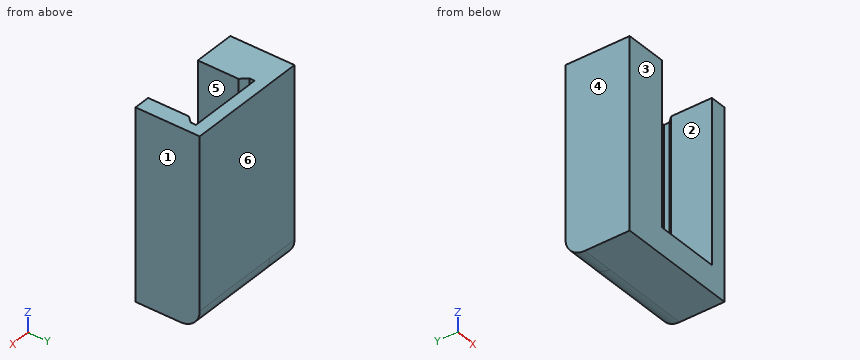
from build123d import *

# Parameters (mm, degrees)
SKETCH_1_W          = 29.5
SKETCH_1_H          = 10
EXTRUDE_1_DEPTH     = 13.06
FILLET_1_R          = 3
CUT_EXTRUDE_1_DEPTH = 25.35
EXTRUDE_START       = 1
EXTRUDE_2_DEPTH     = 1
EXTRUDE_START_2     = -13.06
EXTRUDE_3_DEPTH     = 5


with BuildPart() as part:
    # 草图1 → 凸台-拉伸1 (new body)
    with BuildSketch(Plane(origin=(0, 0, 0), x_dir=(0, 0, -1), z_dir=(1, 0, 0))):
        Rectangle(SKETCH_1_W, SKETCH_1_H)
    extrude(amount=EXTRUDE_1_DEPTH)

    # 圆角1
    fillet_1_edges = [part.edges().sort_by_distance(p)[0] for p in [
        (6.53, 5, -14.75),
    ]]
    fillet(fillet_1_edges, radius=FILLET_1_R)

    # 草图3 → 切除-拉伸1 (cut)
    with BuildSketch(Plane.XY.offset(14.75)):
        Polygon((11.53, -7.004935671), (1.53, -7.004935671), (1.53, 1.342439599), (0.63, 2.342439599), (0.63, 3.15), (12.43, 3.15), (12.43, 2.342439599), (11.53, 1.342439599), align=None)
    extrude(amount=-CUT_EXTRUDE_1_DEPTH, mode=Mode.SUBTRACT)

    # 草图4 → 凸台-拉伸2 (add)
    with BuildSketch(Plane(origin=(13.06, 0, 0), x_dir=(0, 0, -1), z_dir=(1, 0, 0)).offset(EXTRUDE_START)):
        with BuildLine():
            Line((14.75, -5), (14.75, 2))
            ThreePointArc((14.75, 2), (13.871320344, 4.121320344), (11.75, 5))
            Line((11.75, 5), (-14.75, 5))
            Line((-14.75, 5), (-14.75, -5))
            Line((-14.75, -5), (14.75, -5))
        make_face()
    extrude(amount=-EXTRUDE_2_DEPTH)

    # 草图4<3> → 凸台-拉伸3 (add)
    with BuildSketch(Plane(origin=(13.06, 0, 0), x_dir=(0, 0, -1), z_dir=(1, 0, 0)).offset(EXTRUDE_START_2)):
        with BuildLine():
            Line((14.75, -5), (14.75, 2))
            ThreePointArc((14.75, 2), (13.871320344, 4.121320344), (11.75, 5))
            Line((11.75, 5), (-14.75, 5))
            Line((-14.75, 5), (-14.75, -5))
            Line((-14.75, -5), (14.75, -5))
        make_face()
    extrude(amount=-EXTRUDE_3_DEPTH)


solid = part.part
The listing builds one solid part. Answer for the finished solid, in the listing's coordinates (mm). Face numbers are marked on the shaded views. A direction names the side the tool comes from. Coordinates: 2 decimals unless noted, no trailing zeros. Loops run counter-clockwise (first coordinate to the right, second up) from the corner with the lowest first, then second, coordinate; pieces in that order, holes last. Notation, with made-up numbers: (65, 45.5) -> (103, 45.5) arc R21 cw to (103, 84.5) -> close; hole circle Ø5 at (75.25, -28). An arc over 180 degrees is marked (long way). Answer in a Markdown table with one row per item. Add a question column.
1. The part is cut by section D-D, the plane y = 4. Write down the section's boundary in (x, z), then the cut area to 3 significant figures.
2. The part is cut by section C-C, the plane y = -1.25. Write down the section's boundary in (x, z).
3. Determine the mould class of the marked faces 1, 2, 3 and 4 for opening direction X: +X half, -X half, draft (parallel to the pull), parting line (faces both ways), or undercut.
4. Flat-ended cylindrical pins translate along their axes: P1, Ø2, axis at x = 7.5, z = -7, coming from the -Y side; P2, Ø4, axis at x = 7, y = -2, coming from the +Z side. Find the tip coordinate at first contact, or state that the pin passes through.
5. Consider line 1 (Z direction, x = 11, y = -1); line 2 (X direction, y = 1.5, z = 3.5); line 3 (Y direction, x = 10.5, z = -5.25). Determine where each line is inside the solid, lowest interval first. Write a range as [from, to].
6. The part is cut by section A-A, the plane x = 10. Write down the section's boundary in (y, z), then the cut area to 3 significant figures.
7. The part is cut by section B-B, the plane z = 10.25. Write down the section's boundary in (x, y), then the cut area to 3 significant figures.
8. For the marked faces 5 and 6, determine the directions among +Z, -Z, +X, -X, +Y, -Y from which every point of the face is accessible in a straight line to the end or side of a thin tool.
Answer below:
| question | item | result |
|---|---|---|
| 1 | outline | (-5, -13.99) -> (14.06, -13.99) -> (14.06, 14.75) -> (-5, 14.75) -> close |
| 1 | area | 548 mm2 |
| 2 | outline | (-5, -14.75) -> (14.06, -14.75) -> (14.06, 14.75) -> (11.53, 14.75) -> (11.53, -10.6) -> (1.53, -10.6) -> (1.53, 14.75) -> (-5, 14.75) -> close |
| 3 | face 1 | +X half |
| 3 | face 2 | undercut |
| 3 | face 3 | draft |
| 3 | face 4 | -X half |
| 4 | P1 | y = 3.15 |
| 4 | P2 | z = -10.6 |
| 5 | line 1 | [-14.75, -10.6] |
| 5 | line 2 | [-5, 1.39], [11.67, 14.06] |
| 5 | line 3 | [3.15, 5] |
| 6 | outline | (-5, -14.75) -> (2, -14.75) arc R3 ccw to (5, -11.75) -> (5, 14.75) -> (3.15, 14.75) -> (3.15, -10.6) -> (-5, -10.6) -> close |
| 6 | area | 86.5 mm2 |
| 7 | outline | (-5, -5) -> (1.53, -5) -> (1.53, 1.34) -> (0.63, 2.34) -> (0.63, 3.15) -> (12.43, 3.15) -> (12.43, 2.34) -> (11.53, 1.34) -> (11.53, -5) -> (14.06, -5) -> (14.06, 5) -> (-5, 5) -> close |
| 7 | area | 107 mm2 |
| 8 | face 5 | +Z, -Y |
| 8 | face 6 | +Z, -Z, +X, -X, +Y |
